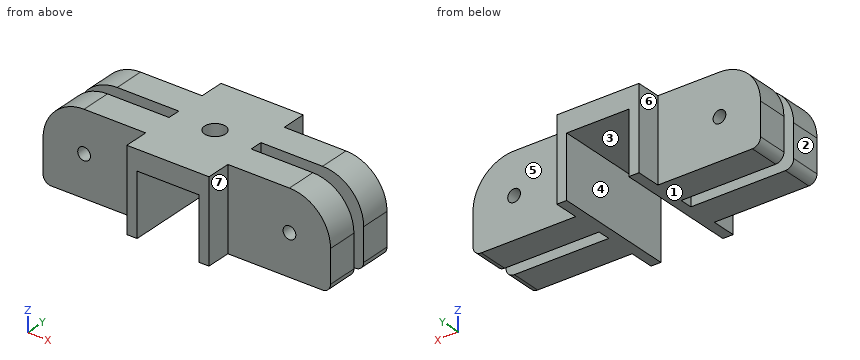
from build123d import *

# Parameters (mm, degrees)
SKETCH_1_R          = 2.55
EXTRUDE_1_DEPTH     = 20
CUT_EXTRUDE_1_REACH = 32
SKETCH_2_W          = 15.1
SKETCH_2_H          = 15.1
SKETCH_3_R          = 1.55
CUT_EXTRUDE_2_DEPTH = 100
FILLET_1_R          = 2
FILLET_2_R          = 10


with BuildPart() as part:
    # 草图1 → 凸台-拉伸1 (new body)
    with BuildSketch(Plane.XY):
        Polygon((10, 9), (10, 15), (-10, 15), (-10, 9), (-35, 9), (-35, 1.55), (-10, 1.55), (-10, -1.55), (-35, -1.55), (-35, -9), (-10, -9), (-10, -15), (10, -15), (10, -9), (35, -9), (35, -1.55), (10, -1.55), (10, 1.55), (35, 1.55), (35, 9), align=None)
        Circle(SKETCH_1_R, mode=Mode.SUBTRACT)
    extrude(amount=EXTRUDE_1_DEPTH)

    # 草图2 → 切除-拉伸1 (cut, up to next)
    with BuildSketch(Plane.XZ.offset(15), mode=Mode.PRIVATE) as cut_extrude_1_sk1:
        with Locations((0.05, 7.55)):
            Rectangle(SKETCH_2_W, SKETCH_2_H)
    cut_extrude_1_tool1 = extrude(cut_extrude_1_sk1.sketch, amount=-CUT_EXTRUDE_1_REACH, mode=Mode.PRIVATE) & part.part
    add(cut_extrude_1_tool1.solids().sort_by_distance((0.05, -15, 7.55))[0], mode=Mode.SUBTRACT)

    # 草图3 → 切除-拉伸2 (cut)
    with BuildSketch(Plane(origin=(0, 9, 0), x_dir=(1, 0, 0), z_dir=(0, 1, 0))):
        with Locations((25, -10)):
            Circle(SKETCH_3_R)
    cut_extrude_2 = extrude(amount=-CUT_EXTRUDE_2_DEPTH, mode=Mode.SUBTRACT)

    # 镜向1: 切除-拉伸2 across plane
    add(cut_extrude_2.mirror(Plane(origin=(0, 0, 0), x_dir=(0, 0, 1), z_dir=(1, 0, 0))), mode=Mode.SUBTRACT)

    # 圆角1
    fillet_1_edges = [part.edges().sort_by_distance(p)[0] for p in [
        (-35, -5.275, 0),
        (-35, 5.275, 0),
        (35, 5.275, 0),
        (35, -5.275, 0),
    ]]
    fillet(fillet_1_edges, radius=FILLET_1_R)

    # 圆角2
    fillet_2_edges = [part.edges().sort_by_distance(p)[0] for p in [
        (35, -5.275, 20),
        (35, 5.275, 20),
        (-35, 5.275, 20),
        (-35, -5.275, 20),
    ]]
    fillet(fillet_2_edges, radius=FILLET_2_R)


solid = part.part
Source: CAD feature listing. Evaluate the final solid. Frame: model axes, mm. Face numbers are marked on the shaded views. A direction names the side the tool comes from. Give positions to 0.01 mm unless a question says otherwise; leave off trailing zeros. Write each loop counter-clockwise with the first axis right and the second up, starting at its lowest first coordinate (ties: lowest second). Pieces come first, ordered by that corner, then holes. Notation, with made-up numbers: M 7.25,24.25 L 19.25,24.25 A14 cw 19.25,51.25 Z; hole C 18.25,-40 d10. An arc over 180 degrees is marked long. Answer as a JSON object with one key per item and string values.
Q1. Ray query, line 1 along X through (y, z) = (-10.25, 1); line 2 along Y through (x, z) = (22.5, 12.75). Return the intervals inside material, ascending.
Geometry check:
{"line 1": "x = -10 to -7.5, 7.6 to 10", "line 2": "y = -9 to -1.55, 1.55 to 9"}
Q2. Cut plane D-D, the plane y = 5. Return the cut outline in (x, z).
Geometry check:
{"outline": "M -35,2 A2 ccw -33,0 L -7.5,0 L -7.5,15.1 L 7.6,15.1 L 7.6,0 L 33,0 A2 ccw 35,2 L 35,10 A10 ccw 25,20 L -25,20 A10 ccw -35,10 Z; hole C -25,10 d3.1; hole C 25,10 d3.1"}
Q3. Cut plane B-B, the plane y = 0. Return the cut outline in (x, z).
Geometry check:
{"outline": "M -10,0 L -7.5,0 L -7.5,15.1 L -2.55,15.1 L -2.55,20 L -10,20 Z; M 2.55,15.1 L 7.6,15.1 L 7.6,0 L 10,0 L 10,20 L 2.55,20 Z"}
Q4. Mould query, pull axis X, two halves, no side actions, for the marked faces 1, 2, 3 and 4. Classes: +X half, -X half, draft (parallel to the pull), parting line (faces both ways), or undercut.
Geometry check:
{"face 1": "draft", "face 2": "-X half", "face 3": "undercut", "face 4": "undercut"}
Q5. Contact query for flat-ended pins moving along their axis: P1, Ø6.5, axis at y = 11, z = 7.5, coming from the +X side; P2, Ø2.5, axis at y = 0, z = 11.5, coming from the -X side; P3, Ø3.5, axis at x = 25, z = 10, coming from the +Y side; P4, Ø3, axis at y = -13.5, z = 7.5, coming from the +X side. Output: stop coordinate, or through.
Geometry check:
{"P1": "stops at x = 35", "P2": "stops at x = -10", "P3": "stops at y = 9", "P4": "stops at x = 10"}
Q6. Access query for the marked faces 5, 6 and 7. Directions: +Z, -Z, +X, -X, +Y, -Y. A direction counts if a zero-diameter tool reaches every point of the face in a straight line with its end or side. Return the directions, or none.
Geometry check:
{"face 5": "+Z, -Z, +X, +Y", "face 6": "+Z, -Z, -X, +Y", "face 7": "+Z, -Z, +X, -Y"}
Q7. Cut plane A-A, the plane x = -14. Return the cut outline in (y, z).
Geometry check:
{"outline": "M -9,0 L -1.55,0 L -1.55,20 L -9,20 Z; M 1.55,0 L 9,0 L 9,20 L 1.55,20 Z"}
Q8. Cut plane C-C, the plane z = 7.75. Return the cut outline in (x, y).
Geometry check:
{"outline": "M -35,-9 L -10,-9 L -10,-15 L -7.5,-15 L -7.5,15 L -10,15 L -10,9 L -35,9 L -35,1.55 L -10,1.55 L -10,-1.55 L -35,-1.55 Z; M 7.6,-15 L 10,-15 L 10,-9 L 35,-9 L 35,-1.55 L 10,-1.55 L 10,1.55 L 35,1.55 L 35,9 L 10,9 L 10,15 L 7.6,15 Z"}
